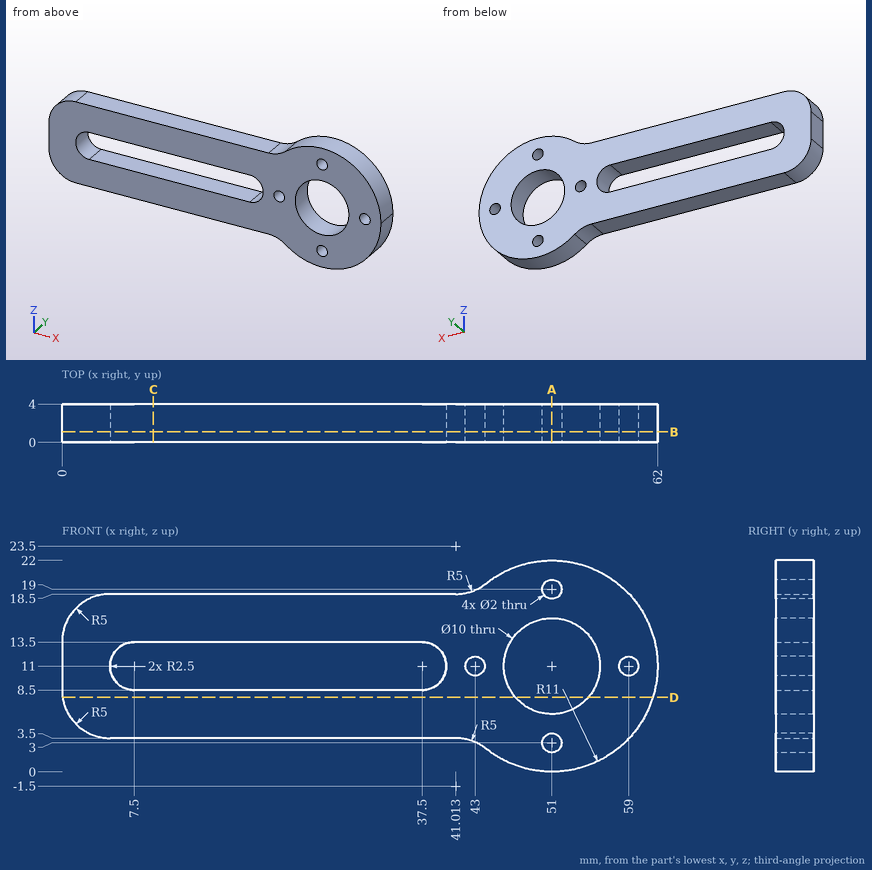
Verification items for this drawing (mm, ordinates from the low corner). Give positions to 0.01 mm unless a question says otherwise; leave off trailing zeros. Write each loop counter-clockwise with the first axis right and the second up, starting at its lowest first coordinate (ties: lowest second). Pieces come first, ordered by that corner, then holes. Notation, with made-up numbers: (41.25, 3) -> (63.25, 3) arc R7 cw to (63.25, 16) -> close; hole circle Ø6 at (83.5, -25.75). An arc over 180 degrees is marked (long way). Use CSV: the item, a comma, the result in double quotes.
(1) Sectioned sample at B-B (y = 1.1). Record the cut outline in (x, z).
Derived:
outline,"(0, 8.5) arc R5 ccw to (5, 3.5) -> (41.01, 3.5) arc R5 cw to (44.13, 2.41) arc R11 ccw to (62, 11) arc R11 ccw to (44.13, 19.59) arc R5 cw to (41.01, 18.5) -> (5, 18.5) arc R5 ccw to (0, 13.5) -> close; hole (7.5, 8.5) -> (37.5, 8.5) arc R2.5 ccw to (37.5, 13.5) -> (7.5, 13.5) arc R2.5 ccw to start; hole circle Ø2 at (43, 11); hole circle Ø10 at (51, 11); hole circle Ø2 at (51, 3); hole circle Ø2 at (51, 19); hole circle Ø2 at (59, 11)"
(2) Sectioned sample at D-D (z = 7.75). Record the cut outline in (x, y).
Derived:
outline,"(0.06, 0) -> (47.2, 0) -> (47.2, 4) -> (0.06, 4) -> close; (54.8, 0) -> (61.51, 0) -> (61.51, 4) -> (54.8, 4) -> close"
(3) Sectioned sample at A-A (x = 51). Record the cut outline in (y, z), plus the area to 3 significant figures.
Derived:
outline,"(0, 0) -> (4, 0) -> (4, 2) -> (0, 2) -> close; (0, 4) -> (4, 4) -> (4, 6) -> (0, 6) -> close; (0, 16) -> (4, 16) -> (4, 18) -> (0, 18) -> close; (0, 20) -> (4, 20) -> (4, 22) -> (0, 22) -> close"
area,"32.0 mm^2"
(4) Sectioned sample at C-C (x = 9.5). Record the cut outline in (y, z), plus the area to 3 significant figures.
Derived:
outline,"(0, 3.5) -> (4, 3.5) -> (4, 8.5) -> (0, 8.5) -> close; (0, 13.5) -> (4, 13.5) -> (4, 18.5) -> (0, 18.5) -> close"
area,"40.0 mm^2"
(5) Material ranges on L1, parallel to Z at x = 51, y = 1.15; L2, parallel to Z at x = 17, y = 3.55; L3, parallel to X at y = 3.85, z = 12.5 (1 decimal), recorded low to high.
Derived:
L1,"z = 0 to 2, 4 to 6, 16 to 18, 20 to 22"
L2,"z = 3.5 to 8.5, 13.5 to 18.5"
L3,"x = 0 to 5.5, 39.5 to 46.2, 55.8 to 61.9"
(6) Go/stop test with flat-tipped pins: pin 1 (1.2 mm diameter, centred on x = 29.5, y = 3, fed in from +Z); pin 2 (2 mm diameter, centred on x = 27, y = 1, fed in from -Z). Record where each tip stops, or that it passes through.
Derived:
pin 1,"stops at z = 18.5"
pin 2,"stops at z = 3.5"
